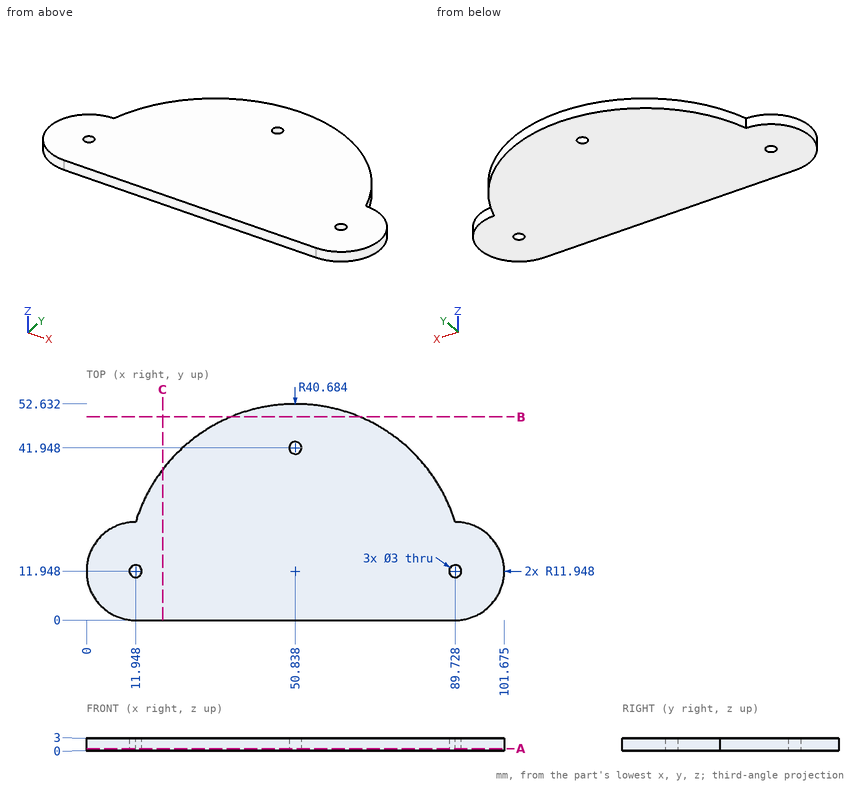
Design review of the part shown in the three views and the two pictorial views. Dimensions are in mm from the part's minimum x, y and z. Coordinates: 2 decimals unless noted, no trailing zeros. Loops run counter-clockwise (first coordinate to the right, second up) from the corner with the lowest first, then second, coordinate; pieces in that order, holes last. Notation, with made-up numbers: (-2, -36.5) - (21, -36.5) arc R37 cw to (21, 0.5) - close; hole circle Ø1 at (89, 52.25). An arc over 180 degrees is marked (long way). Use a Markdown table: item, result. Add a question column.
Item 1: For line 1 (X direction, y = 13, z = 0.35) (1 decimal); line 2 (Y direction, x = 51, z = 2.5); line 3 (Y direction, x = 29.5, z = 1.1) (1 decimal), list the stretches that pass through material, from the lowest coordinate up.
Item 2: Insertion check: pin 1 Ø1 at (y, z) = (38.5, 0.5) entering from +X (1 decimal). The pin has a flat end and moves straight along its axis. Give the tip position at first contact, or say it passes through.
Item 3: We need section A-A (z = 0.45). Give the boundary of the cut face in (x, y) (1 decimal), and give its area (3 significant figures).
Item 4: We need section B-B (y = 49.5). Give the boundary of the cut face in (x, z) (1 decimal).
Item 5: We need section C-C (x = 18.5). Give the boundary of the cut face in (y, z) (1 decimal).
Results list:
| question | item | result |
|---|---|---|
| 1 | line 1 | x = 0 to 10.9, 13 to 88.7, 90.8 to 101.6 |
| 1 | line 2 | y = 0 to 40.46, 43.44 to 52.63 |
| 1 | line 3 | y = 0 to 46.6 |
| 2 | pin 1 | stops at x = 82.1 |
| 3 | outline | (11.9, 0) - (89.7, 0) arc R11.9 ccw to (89.7, 23.9) arc R40.7 ccw to (11.9, 23.9) arc R11.9 ccw to start; hole circle Ø3 at (11.9, 11.9); hole circle Ø3 at (50.8, 41.9); hole circle Ø3 at (89.7, 11.9) |
| 3 | area | 3,930 mm^2 |
| 4 | outline | (35.2, 0) - (66.5, 0) - (66.5, 3) - (35.2, 3) - close |
| 5 | outline | (0, 0) - (36.6, 0) - (36.6, 3) - (0, 3) - close |
